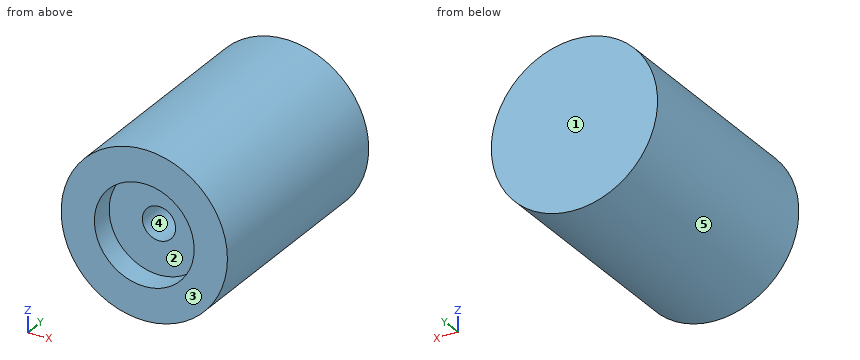
```python
from build123d import *

# Parameters (mm, degrees)
F0_R      = 50
F1_DEPTH  = 70
F1_FACE_R = 50
F2_DEPTH  = 70
F3_R      = 30
F4_DEPTH  = 40
F5_R      = 30
F6_DEPTH  = 25.4
F7_R      = 10
F8_DEPTH  = 80


with BuildPart() as f1:
    # F0 (on Front) → F1 (new body)
    with BuildSketch(Plane.XZ):
        Circle(F0_R)
    extrude(amount=F1_DEPTH)

    # F1_face (on face) → F2 (join)
    with BuildSketch(Plane(origin=(0, 0, 0), x_dir=(1, 0, 0), z_dir=(0, 1, 0))):
        Circle(F1_FACE_R)
    extrude(amount=F2_DEPTH)

    # F3 (on face) → F4 (cut)
    with BuildSketch(Plane.XZ.offset(70)):
        Circle(F3_R)
    extrude(amount=-F4_DEPTH, mode=Mode.SUBTRACT)

    # F5 (on face) → F6 (join)
    with BuildSketch(Plane.XZ.offset(30)):
        Circle(F5_R)
    extrude(amount=F6_DEPTH)

    # F7 (on face) → F8 (cut)
    with BuildSketch(Plane.XZ.offset(55.4)):
        Circle(F7_R)
    extrude(amount=-F8_DEPTH, mode=Mode.SUBTRACT)


solid = f1.part
```
Can you work these out from the model? Positions are in its coordinate system, mm. Face numbers are marked on the shaded views. A direction names the side the tool comes from. Coordinates: 2 decimals unless noted, no trailing zeros. Loops run counter-clockwise (first coordinate to the right, second up) from the corner with the lowest first, then second, coordinate; pieces in that order, holes last. Notation, with made-up numbers: M 76,-19.75 L 125,-19.75 A26 cw 125,-3.75 Z; hole C -24,-12.75 d8. An arc over 180 degrees is marked long. Put each result on its own line as item: value. Start each with the question number.
(1) Which directions (+Z, -Z, +X, -X, +Y, -Y) give clear straight access to the entire face, cutting with the end or side of a thin tool? Please do the marked faces 1 and 2.
(2) Imagine slicing it at A-A on z = 0. List the corners of the cut face in (x, y) for me.
(3) Imagine slicing it at D-D on y = 39. List the corners of the cut face in (x, z) for me.
(4) Imagine slicing it at C-C on y = -2. List the corners of the cut face in (x, z) for me, and give its area (3 significant figures).
(5) I need wall thicknesses on probe 1 along Z at (x, y) = (0, -14); probe 2 along Z at (x, y) = (0, -62); probe 3 along Y at (x, z) = (-6, -3.5). Which ranges of each line are inside material? Lowest first, please.
(6) Will these pins go through, and if not, where does the flat tip stop? pin 1 Ø12 at (x, y) = (-1, 33) entering from +Z; pin 2 Ø22 at (x, z) = (-3, 1) entering from -Y; pin 3 Ø5 at (x, y) = (30.5, 9) entering from +Z.
(7) We'd pull the mould along Z, two halves only. Please class the marked faces 3, 4 and 5: +Z half, -Z half, draft (parallel to the pull), parting line (faces both ways), or undercut.
(8) Imagine slicing it at B-B on x = 0. List the corners of the cut face in (y, z) for me.
Worked answers:
1. face 1: +Z, -Z, +X, -X, +Y
1. face 2: -Y
2. outline: M -50,-70 L -30,-70 L -30,-55.4 L -10,-55.4 L -10,24.6 L 10,24.6 L 10,-55.4 L 30,-55.4 L 30,-70 L 50,-70 L 50,70 L -50,70 Z
3. outline: C 0,0 d100
4. outline: C 0,0 d100; hole C 0,0 d20
4. area: 7,540 mm2
5. probe 1: z = -50 to -10, 10 to 50
5. probe 2: z = -50 to -30, 30 to 50
5. probe 3: y = 24.6 to 70
6. pin 1: stops at z = 50
6. pin 2: stops at y = -55.4
6. pin 3: stops at z = 41.42
7. face 3: draft
7. face 4: undercut
7. face 5: parting line
8. outline: M -70,-50 L 70,-50 L 70,50 L -70,50 L -70,30 L -55.4,30 L -55.4,10 L 24.6,10 L 24.6,-10 L -55.4,-10 L -55.4,-30 L -70,-30 Z
